```python
from build123d import *

# Parameters (mm, degrees)
ESQUISSE1_R        = 32
BOSS_EXTRU_1_DEPTH = 100
BOSS_EXTRU_1_DRAFT = -3
COQUE3_T           = 2
CONG_7_R           = 2


with BuildPart() as part:
    # Esquisse1 → Boss.-Extru.1 (with draft: the straight prism first)
    with BuildSketch(Plane.XY):
        Circle(ESQUISSE1_R)
    extrude(amount=BOSS_EXTRU_1_DEPTH)
    # Boss.-Extru.1: the draft: its side faces are tilted about the plane it starts from
    boss_extru_1_sides = [part.faces().sort_by_distance(p)[0] for p in [
        (-32, 0, 50),
    ]]
    draft(boss_extru_1_sides, Plane.XY, BOSS_EXTRU_1_DRAFT)

    # Coque3
    coque3_openings = [part.faces().sort_by_distance(p)[0] for p in [
        (0, 0, 100),
    ]]
    offset(amount=COQUE3_T, openings=coque3_openings, kind=Kind.INTERSECTION)

    # Congé6: read off the stored shape, not the designer's step
    # Congé6 outline → Congé6 (revolve, cut)
    with BuildSketch(Plane.XZ):
        with BuildLine():
            ThreePointArc((34.146253974, 2.738320219), (32.594879178, -0.626871855), (29.1531063, -2))
            Line((29.1531063, -2), (34.146253974, -2))
            Line((34.146253974, -2), (34.146253974, 2.738320219))
        make_face()
    revolve(axis=Axis((0, 0, 0), (0, 0, 1)), mode=Mode.SUBTRACT)

    # Congé7
    # the kernel refuses this fillet: 2 mm, written as the material it takes off along each edge
    with BuildSketch(Plane(origin=(0, 0, 100), x_dir=(1, 0, 0), z_dir=(0, 1, 0))) as cong_7_piece_1:
        with BuildLine():
            CenterArc((37.136106016, 1.99725907), CONG_7_R, 273, 90)
            Line((39.133365085, 2.101930982), (39.173310267, 2.10402442))
            Line((39.173310267, 2.10402442), (39.283467802, 0.002093438))
            Line((39.283467802, 0.002093438), (39.24352262, -0.04))
            ThreePointArc((39.24352262, -0.04), (38.242150274, -0.04), (37.242871367, -0.039945181))
            Line((37.242871367, -0.039945181), (37.240777928, 0))
        make_face()
    revolve(axis=Axis((0, 0, 100), (0, 0, -1)), mode=Mode.SUBTRACT)


solid = part.part
```
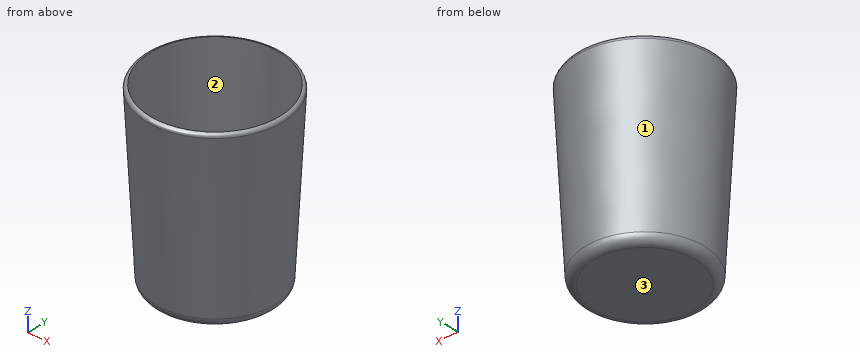
Could you check a few things on this model? Use its own coordinates, in mm. Face numbers are marked on the shaded views. Coordinates: 2 decimals unless noted, no trailing zeros. Write each loop counter-clockwise with the first axis right and the second up, starting at its lowest first coordinate (ties: lowest second). Pieces come first, ordered by that corner, then holes. Notation, with made-up numbers: (-34.75, 63) -> (1.25, 63) arc R16 cw to (1.25, 77) -> close; hole circle Ø1 at (40, 38.5). An arc over 180 degrees is marked (long way). Write item = value, one per line. Start each with the question number.
(1) I want a section at D-D (z = 56.5). Please give me the cut outline in (x, y).
(2) I want a section at A-A (x = 0). Please give me the cut outline in (y, z).
(3) I want a section at C-C (z = 80). Please give me the cut outline in (x, y).
(4) We'd pull the mould along Y, two halves only. Please class the marked faces 1, 2 and 3: released by +Y, released by -Y, zero draft, split by the parting line, or undercut.
(5) I need wall thicknesses on line 1 (Z direction, x = -12, y = -25.5); line 2 (Y direction, x = -14.5, z = 24); line 3 (Y direction, x = -16, z = 24). Which ranges of each line are inside material? Lowest first, please. Write a range as [from, to].
(6) Will these pins go through, and if not, where does the flat tip stop? pin 1 (10 mm diameter, centred on y = -29.5, z = 44.5, fed in from -X); pin 2 (12 mm diameter, centred on x = 3.5, z = 15, fed in from +Y); pin 3 (1 mm diameter, centred on x = 31, y = -13.5, fed in from -Z).
Result set:
q1.outline = circle Ø73.93 at (0, 0); hole circle Ø69.92 at (0, 0)
q2.outline = (-39.13, 97.9) -> (-34.15, 2.74) arc R5 ccw to (-29.15, -2) -> (29.15, -2) arc R5 ccw to (34.15, 2.74) -> (39.13, 97.9) arc R2 ccw to (37.24, 100) -> (32, 0) -> (-32, 0) -> (-37.24, 100) arc R2 ccw to start
q3.outline = circle Ø76.39 at (0, 0); hole circle Ø72.39 at (0, 0)
q4.face_1 = split by the parting line
q4.face_2 = undercut
q4.face_3 = zero draft
q5.line_1 = [-2, 0]
q5.line_2 = [-32.14, -29.93], [29.93, 32.14]
q5.line_3 = [-31.42, -29.16], [29.16, 31.42]
q6.pin_1 = -26.85
q6.pin_2 = 35.06
q6.pin_3 = 0.22
